Could you check a few things on this model? Use its own coordinates, in mm. Face numbers are marked on the shaded views. A direction names the side the tool comes from. Round coordinates to 2 decimals unless told otherwise and drop trailing zeros. Order: outer loops, then holes, each group sorted by start corner. A loop starts at its lowest first (then second) coordinate and runs counter-clockwise, first axis right, second up. Notation, with made-up numbers: (-22.5, -13) - (21.5, -13) arc R14 cw to (21.5, 1) - close; hole circle Ø2 at (-23.75, 55.25). An arc over 180 degrees is marked (long way). Use one line per item in the form item = value.
from build123d import *

# Parameters (mm, degrees)
SKETCH1_W            = 90
SKETCH1_H            = 80
BOSS_EXTRUDE1_DEPTH  = 3
SKETCH2_W            = 11.75
SKETCH2_H            = 50
CUT_EXTRUDE1_DEPTH   = 3
SKETCH3_W            = 2
SKETCH3_H            = 15
BOSS_EXTRUDE2_DEPTH  = 3
BOSS_EXTRUDE3_DEPTH  = 3
CUT_EXTRUDE2_DEPTH   = 3
BOSS_EXTRUDE4_DEPTH  = 45
BOSS_EXTRUDE5_DEPTH  = 3
CUT_EXTRUDE3_DEPTH   = 3
CUT_EXTRUDE6_START   = -93.59401
CUT_EXTRUDE6_DEPTH   = 93.644295
MIRROR4_START        = 35.25
MIRROR4_DEPTH        = 11.572147393
SKETCH17_W           = 70.5
SKETCH17_H           = 3
BOSS_EXTRUDE10_DEPTH = 3
SKETCH19_W           = 79.626439034
SKETCH19_H           = 3
BOSS_EXTRUDE11_DEPTH = 10
CUT_EXTRUDE7_DEPTH   = 10
SKETCH22_W           = 87.543724768
SKETCH22_H           = 9.2
BOSS_EXTRUDE12_DEPTH = 3
CUT_EXTRUDE8_DEPTH   = 5
CUT_EXTRUDE9_DEPTH   = 5
FILLET4_R            = 1.5
FILLET6_R            = 1.5
SKETCH26_W           = 20
SKETCH26_H           = 10
CUT_EXTRUDE10_DEPTH  = 5


# Read off the part's stored shape, not the designer's step: Mirror4
with BuildPart() as part:
    # Sketch1 → Boss-Extrude1 (new body)
    with BuildSketch(Plane(origin=(0, 0, 0), x_dir=(1, 0, 0), z_dir=(0, 1, 0))):
        Rectangle(SKETCH1_W, SKETCH1_H)
    extrude(amount=BOSS_EXTRUDE1_DEPTH)

    # Sketch2 → Cut-Extrude1 (cut)
    with BuildSketch(Plane(origin=(0, 3, 0), x_dir=(1, 0, 0), z_dir=(0, 1, 0))):
        with Locations((-39.125, 0)):
            Rectangle(SKETCH2_W, SKETCH2_H)
        with Locations((39.125, 0)):
            Rectangle(SKETCH2_W, SKETCH2_H)
    extrude(amount=-CUT_EXTRUDE1_DEPTH, mode=Mode.SUBTRACT)

    # Sketch3 → Boss-Extrude2 (add)
    with BuildSketch(Plane(origin=(0, 3, 0), x_dir=(1, 0, 0), z_dir=(0, 1, 0))):
        with Locations((-34.25, -17.5)):
            Rectangle(SKETCH3_W, SKETCH3_H)
        with Locations((-34.25, 17.5)):
            Rectangle(SKETCH3_W, SKETCH3_H)
        with Locations((34.25, -17.5)):
            Rectangle(SKETCH3_W, SKETCH3_H)
        with Locations((34.25, 17.5)):
            Rectangle(SKETCH3_W, SKETCH3_H)
    extrude(amount=-BOSS_EXTRUDE2_DEPTH)

    # Sketch4 → Boss-Extrude3 (add)
    with BuildSketch(Plane(origin=(0, 3, 0), x_dir=(1, 0, 0), z_dir=(0, 1, 0))):
        Polygon((-45, 25), (-46.822147393, 25), (-45, 30.668057955), align=None)
        Polygon((45, 25), (46.822147393, 25), (45, 30.668057955), align=None)
        Polygon((-45, -25), (-46.822147393, -25), (-45, -30.668057955), align=None)
        Polygon((45, -25), (46.822147393, -25), (45, -30.668057955), align=None)
    extrude(amount=-BOSS_EXTRUDE3_DEPTH)

    # Sketch5 → Cut-Extrude2 (cut)
    with BuildSketch(Plane(origin=(0, 3, 0), x_dir=(1, 0, 0), z_dir=(0, 1, 0))):
        Polygon((-45, 30.668057955), (-42, 40), (-45, 40), align=None)
        Polygon((45, 30.668057955), (42, 40), (45, 40), align=None)
        Polygon((45, -40), (45, -30.668057955), (42, -40), align=None)
        Polygon((-45, -40), (-45, -30.668057955), (-42, -40), align=None)
    extrude(amount=-CUT_EXTRUDE2_DEPTH, mode=Mode.SUBTRACT)

    # Sketch6 → Boss-Extrude4 (add)
    with BuildSketch(Plane(origin=(0, 3, 0), x_dir=(1, 0, 0), z_dir=(0, 1, 0))):
        Polygon((39.813219517, 37), (-39.813219517, 37), (-43.670937432, 25), (-46.822147393, 25), (-42, 40), (42, 40), (46.771862384, 25.156418928), (46.771862384, 25), (43.670937432, 25), align=None)
        Polygon((43.670937432, -25), (39.813219517, -37), (-39.813219517, -37), (-43.670937432, -25), (-46.822147393, -25), (-42, -40), (42, -40), (46.822147393, -25), align=None)
    extrude(amount=BOSS_EXTRUDE4_DEPTH)

    # Sketch7 → Boss-Extrude5 (add)
    with BuildSketch(Plane(origin=(46.771862384, 0, 0), x_dir=(0, 0, -1), z_dir=(1, 0, 0))):
        with BuildLine():
            Line((-25, 25.5), (-25, 48))
            Line((-25, 48), (25.156418928, 48))
            Line((25.156418928, 48), (25.156418928, 25.5))
            ThreePointArc((25.156418928, 25.5), (0.078209464, 38.896159305), (-25, 25.5))
        make_face()
    boss_extrude5 = extrude(amount=-BOSS_EXTRUDE5_DEPTH)

    # Mirror1: Boss-Extrude5 across plane
    add(boss_extrude5.mirror(Plane.ZY))

    # Sketch10 → Cut-Extrude3 (cut)
    with BuildSketch(Plane(origin=(0, 0, -40), x_dir=(-1, 0, 0), z_dir=(0, 0, -1))):
        with BuildLine():
            Line((-12.5, 23), (12.5, 23))
            ThreePointArc((12.5, 23), (20.5, 15), (12.5, 7))
            Line((12.5, 7), (-12.5, 7))
            ThreePointArc((-12.5, 7), (-20.5, 15), (-12.5, 23))
        make_face()
    extrude(amount=-CUT_EXTRUDE3_DEPTH, mode=Mode.SUBTRACT)

    # Sketch15 → Cut-Extrude6 (cut)
    with BuildSketch(Plane(origin=(46.771862384, 0, 0), x_dir=(0, 0, -1), z_dir=(1, 0, 0)).offset(CUT_EXTRUDE6_START)):
        Polygon((25, 25.731506228), (25, 0), (28, 0), align=None)
    cut_extrude6 = extrude(amount=CUT_EXTRUDE6_DEPTH, mode=Mode.SUBTRACT)

    # Mirror3: Cut-Extrude6 across plane
    add(cut_extrude6.mirror(Plane.ZY), mode=Mode.SUBTRACT)

    # Mirror4 outline → Mirror4 (cut)
    with BuildSketch(Plane.YZ.offset(MIRROR4_START)):
        Polygon((25.731506228, 25), (0, 28), (0, 25), align=None)
    extrude(amount=MIRROR4_DEPTH, mode=Mode.SUBTRACT)

    # Sketch17 → Boss-Extrude10 (add)
    with BuildSketch(Plane(origin=(0, 0, -25), x_dir=(-1, 0, 0), z_dir=(0, 0, -1))):
        with Locations((0, 1.5)):
            Rectangle(SKETCH17_W, SKETCH17_H)
    extrude(amount=BOSS_EXTRUDE10_DEPTH)

    # Sketch19 → Boss-Extrude11 (add)
    with BuildSketch(Plane(origin=(0, 0, 37), x_dir=(-1, 0, 0), z_dir=(0, 0, -1))):
        with Locations((0, 31.5)):
            Rectangle(SKETCH19_W, SKETCH19_H)
    extrude(amount=BOSS_EXTRUDE11_DEPTH)

    # Sketch21 → Cut-Extrude7 (cut)
    with BuildSketch(Plane(origin=(0, 33, 0), x_dir=(1, 0, 0), z_dir=(0, 1, 0))):
        with BuildLine():
            Line((-34.155163783, -30.4), (32.512648359, -30.4))
            ThreePointArc((32.512648359, -30.4), (34.112648359, -32), (32.512648359, -33.6))
            Line((32.512648359, -33.6), (-34.155163783, -33.6))
            ThreePointArc((-34.155163783, -33.6), (-35.755163783, -32), (-34.155163783, -30.4))
        make_face()
    extrude(amount=-CUT_EXTRUDE7_DEPTH, mode=Mode.SUBTRACT)

    # Sketch22 → Boss-Extrude12 (add)
    with BuildSketch(Plane(origin=(0, 33, 0), x_dir=(1, 0, 0), z_dir=(0, 1, 0))):
        with Locations((0, 23.2)):
            Rectangle(SKETCH22_W, SKETCH22_H)
        with BuildLine():
            Line((-34.528137616, 24.8), (35.471862384, 24.8))
            ThreePointArc((35.471862384, 24.8), (37.071862384, 23.2), (35.471862384, 21.6))
            Line((35.471862384, 21.6), (-34.528137616, 21.6))
            ThreePointArc((-34.528137616, 21.6), (-36.128137616, 23.2), (-34.528137616, 24.8))
        make_face(mode=Mode.SUBTRACT)
    extrude(amount=-BOSS_EXTRUDE12_DEPTH)

    # Sketch24 → Cut-Extrude8 (cut)
    with BuildSketch(Plane.ZY.offset(43.771862384)):
        Polygon((-18.6, 32.542028326), (-18.6, 30), (-21.471793131, 30), align=None)
    extrude(amount=-CUT_EXTRUDE8_DEPTH, mode=Mode.SUBTRACT)

    # Sketch25 → Cut-Extrude9 (cut)
    with BuildSketch(Plane(origin=(43.771862384, 0, 0), x_dir=(0, 0, -1), z_dir=(1, 0, 0))):
        Polygon((18.6, 32.542028326), (18.6, 30), (21.471793131, 30), align=None)
    extrude(amount=-CUT_EXTRUDE9_DEPTH, mode=Mode.SUBTRACT)

    # Fillet4
    fillet4_edges = [part.edges().sort_by_distance(p)[0] for p in [
        (38.771862384, 31.271014163, -20.035896565),
    ]]
    fillet(fillet4_edges, radius=FILLET4_R)

    # Fillet6
    fillet6_edges = [part.edges().sort_by_distance(p)[0] for p in [
        (-38.771862384, 31.271014163, -20.035896565),
    ]]
    fillet(fillet6_edges, radius=FILLET6_R)

    # Sketch26 → Cut-Extrude10 (cut)
    with BuildSketch(Plane(origin=(0, 0, 37), x_dir=(-1, 0, 0), z_dir=(0, 0, -1))):
        with Locations((-0.186780483, 43)):
            Rectangle(SKETCH26_W, SKETCH26_H)
    extrude(amount=-CUT_EXTRUDE10_DEPTH, mode=Mode.SUBTRACT)


solid = part.part
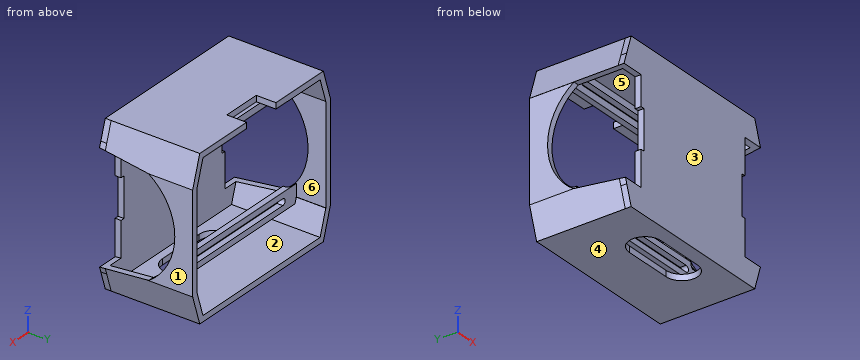
Item 1: If we mould it in two halves opening along X, with no side actions, what happens to the marked faces 1, 2 and 3? For each: released by +X, released by -X, zero draft, split by the parting line, or undercut.
Found:
face_1 = released by +X
face_2 = undercut
face_3 = zero draft
Item 2: Will these pins go through, and if not, where does the flat tip stop? P1, Ø1.5, axis at y = 1.5, z = -3, coming from the +X side; P2, Ø0.9, axis at y = 2, z = 23, coming from the +X side; P3, Ø7.5, axis at x = -8.5, z = -21.5, coming from the -Y side; P4, Ø12, axis at x = -15.5, z = -1, coming from the +Y side.
Found:
P1 = 33.25
P2 = 35.25
P3 = 0
P4 = 3
Item 3: Imagine slicing it at C-C on y = 11. Please give me the cut outline in (x, z), plus the area to 3 significant figures.
Found:
outline = (-46.82, 25) - (-43.67, 25) - (-39.81, 37) - (39.81, 37) - (43.12, 26.72) - (46.27, 26.72) - (42, 40) - (-42, 40) - close; (-46.27, -26.72) - (-42, -40) - (-19.43, -40) - (-19.43, -37) - (-39.81, -37) - (-43.12, -26.72) - close; (19.43, -40) - (42, -40) - (46.27, -26.72) - (43.12, -26.72) - (39.81, -37) - (19.43, -37) - close
area = 528 mm2
Item 4: For the marked faces 4, 5 and 6, which set-ups out of +Z, -Z, +X, -X, +Y, -Y let a thin tool reach every point of the face, with its end or its side?
Found:
face_4 = -Z, +X, -X, +Y, -Y
face_5 = none
face_6 = +Y
Item 5: Imagine slicing it at B-B on z = 14. Please give me the cut outline in (x, y).
Found:
outline = (-46.77, 35.41) - (-43.77, 35.41) - (-43.77, 48) - (-46.77, 48) - close; (-35.25, 0) - (35.25, 0) - (35.25, 3) - (-35.25, 3) - close; (43.77, 35.41) - (46.77, 35.41) - (46.77, 48) - (43.77, 48) - close
Item 6: I need wall thicknesses on L1, parallel to X at y = 36, z = 19; L2, parallel to Z at x = 30.5, y = 16.5; L3, parallel to Y at x = -25, z = -19. Which ranges of each line are inside material? Lowest first, please.
Found:
L1 = -46.77 to -43.77, 43.77 to 46.77
L2 = -40 to -37, 37 to 40
L3 = 0 to 3, 30 to 33
Item 7: Imagine slicing it at A-A on x = 1. Please give me the cut outline in (y, z), plus the area to 3 significant figures.
Found:
outline = (0, -40) - (7, -40) - (7, -37) - (3, -37) - (3, 37) - (30, 37) - (30, 33.6) - (33, 33.6) - (33, 37) - (38, 37) - (38, 40) - (0, 40) - close; (23, -40) - (48, -40) - (48, -37) - (23, -37) - close; (30, -27.8) - (33, -27.8) - (33, -24.8) - (30, -24.8) - close; (30, -21.6) - (33, -21.6) - (33, -18.6) - (30, -18.6) - close; (30, 27) - (33, 27) - (33, 30.4) - (30, 30.4) - close
area = 470 mm2
Item 8: Imagine slicing it at D-D on x = -18. Please give me the cut outline in (y, z).
Found:
outline = (0, -40) - (9.19, -40) - (9.19, -37) - (3, -37) - (3, 37) - (30, 37) - (30, 33.6) - (33, 33.6) - (33, 37) - (48, 37) - (48, 40) - (0, 40) - close; (20.81, -40) - (48, -40) - (48, -37) - (20.81, -37) - close; (30, -27.8) - (33, -27.8) - (33, -24.8) - (30, -24.8) - close; (30, -21.6) - (33, -21.6) - (33, -18.6) - (30, -18.6) - close; (30, 27) - (33, 27) - (33, 30.4) - (30, 30.4) - close
